Verification items for the finished model (mm, model axes). A direction names the side the tool comes from. Give positions to 0.01 mm unless a question says otherwise; leave off trailing zeros. Order: outer loops, then holes, each group sorted by start corner. A loop starts at its lowest first (then second) coordinate and runs counter-clockwise, first axis right, second up.
from build123d import *

# Parameters (mm, degrees)
BLOCK_BODY_DEPTH                       = 19.7
SIDE_REFERENCE_SKETCH_W                = 40
SIDE_REFERENCE_SKETCH_H                = 20
SIDE_REFERENCE_DEPTH                   = 0.45
AESTHETIC_CHAMFER_1_SIZE               = 0.5
CASTING_GROOVE_SKETCH_W                = 6
CASTING_GROOVE_SKETCH_H                = 40
CASTING_GOORVE_DEPTH                   = 0.75
AESTHETIC_CHAMFER_2_SIZE               = 0.2
PRODUCTION_FILLET_R                    = 0.2
FIXING_HOLES_D                         = 3.3
FIXING_HOLES_DEPTH                     = 7.1
FIXING_HOLES_CSINK_D                   = 4.2
FIXING_HOLES_CSINK_ANGLE               = 90
FIXING_HOLES_TIP                       = 0.991420021
END_CAP_FIXING_HOLES_FRONT_D           = 2.05
END_CAP_FIXING_HOLES_FRONT_DEPTH       = 6.35
END_CAP_FIXING_HOLES_FRONT_CSINK_D     = 2.7
END_CAP_FIXING_HOLES_FRONT_CSINK_ANGLE = 90
END_CAP_FIXING_HOLES_FRONT_TIP         = 0.615882135
END_CAP_FIXING_HOLES_BACK_D            = 2.05
END_CAP_FIXING_HOLES_BACK_DEPTH        = 6.35
END_CAP_FIXING_HOLES_BACK_CSINK_D      = 2.7
END_CAP_FIXING_HOLES_BACK_CSINK_ANGLE  = 90
END_CAP_FIXING_HOLES_BACK_TIP          = 0.615882135


with BuildPart() as part:
    # Block Profile → Block Body (new body, symmetric)
    with BuildSketch(Plane.XY):
        with BuildLine():
            Line((16, 4.3), (13, 4.3))
            Line((13, 4.3), (13, 8.2))
            ThreePointArc((13, 8.2), (12.970710678, 8.270710678), (12.9, 8.3))
            Line((12.9, 8.3), (4.85, 8.3))
            Line((4.85, 8.3), (4.85, 8.584314575))
            ThreePointArc((4.85, 8.584314575), (4.87283614, 8.699119605), (4.937867966, 8.796446609))
            Line((4.937867966, 8.796446609), (5.13367604, 8.992254684))
            ThreePointArc((5.13367604, 8.992254684), (5.223715255, 9.115101334), (5.272591987, 9.259356056))
            ThreePointArc((5.272591987, 9.259356056), (5.689339828, 10.060660172), (6.490643944, 10.477408013))
            ThreePointArc((6.490643944, 10.477408013), (6.766607459, 10.625414027), (6.900414725, 10.908534598))
            ThreePointArc((6.900414725, 10.908534598), (6.98601637, 11.08386098), (7.161342753, 11.169462626))
            ThreePointArc((7.161342753, 11.169462626), (7.474614052, 11.334529402), (7.6, 11.665685425))
            Line((7.6, 11.665685425), (7.6, 12.334314575))
            ThreePointArc((7.6, 12.334314575), (7.474614052, 12.665470598), (7.161342753, 12.830537374))
            ThreePointArc((7.161342753, 12.830537374), (6.98601637, 12.91613902), (6.900414725, 13.091465402))
            ThreePointArc((6.900414725, 13.091465402), (6.766607459, 13.374585973), (6.490643944, 13.522591987))
            ThreePointArc((6.490643944, 13.522591987), (5.689339828, 13.939339828), (5.272591987, 14.740643944))
            ThreePointArc((5.272591987, 14.740643944), (5.223715255, 14.884898666), (5.13367604, 15.007745316))
            Line((5.13367604, 15.007745316), (5.041421356, 15.1))
            Line((5.041421356, 15.1), (-5.041421356, 15.1))
            Line((-5.041421356, 15.1), (-5.13367604, 15.007745316))
            ThreePointArc((-5.13367604, 15.007745316), (-5.223715255, 14.884898666), (-5.272591987, 14.740643944))
            ThreePointArc((-5.272591987, 14.740643944), (-5.689339828, 13.939339828), (-6.490643944, 13.522591987))
            ThreePointArc((-6.490643944, 13.522591987), (-6.766607459, 13.374585973), (-6.900414725, 13.091465402))
            ThreePointArc((-6.900414725, 13.091465402), (-6.98601637, 12.91613902), (-7.161342753, 12.830537374))
            ThreePointArc((-7.161342753, 12.830537374), (-7.474614052, 12.665470598), (-7.6, 12.334314575))
            Line((-7.6, 12.334314575), (-7.6, 11.665685425))
            ThreePointArc((-7.6, 11.665685425), (-7.474614052, 11.334529402), (-7.161342753, 11.169462626))
            ThreePointArc((-7.161342753, 11.169462626), (-6.98601637, 11.08386098), (-6.900414725, 10.908534598))
            ThreePointArc((-6.900414725, 10.908534598), (-6.766607459, 10.625414027), (-6.490643944, 10.477408013))
            ThreePointArc((-6.490643944, 10.477408013), (-5.689339828, 10.060660172), (-5.272591987, 9.259356056))
            ThreePointArc((-5.272591987, 9.259356056), (-5.223715255, 9.115101334), (-5.13367604, 8.992254684))
            Line((-5.13367604, 8.992254684), (-4.937867966, 8.796446609))
            ThreePointArc((-4.937867966, 8.796446609), (-4.87283614, 8.699119605), (-4.85, 8.584314575))
            Line((-4.85, 8.584314575), (-4.85, 8.3))
            Line((-4.85, 8.3), (-12.9, 8.3))
            ThreePointArc((-12.9, 8.3), (-12.970710678, 8.270710678), (-13, 8.2))
            Line((-13, 8.2), (-13, 4.3))
            Line((-13, 4.3), (-16, 4.3))
            Line((-16, 4.3), (-17, 5.3))
            Line((-17, 5.3), (-17, 27))
            Line((-17, 27), (-16, 28))
            Line((-16, 28), (16, 28))
            Line((16, 28), (17, 27))
            Line((17, 27), (17, 5.3))
            Line((17, 5.3), (16, 4.3))
        make_face()
    extrude(amount=BLOCK_BODY_DEPTH, both=True)

    # Side Reference Sketch → Side Reference (cut)
    with BuildSketch(Plane(origin=(17, 0, 0), x_dir=(0, 0, -1), z_dir=(1, 0, 0))):
        with Locations((0, 12)):
            Rectangle(SIDE_REFERENCE_SKETCH_W, SIDE_REFERENCE_SKETCH_H)
    extrude(amount=-SIDE_REFERENCE_DEPTH, mode=Mode.SUBTRACT)

    # Aesthetic Chamfer 1
    aesthetic_chamfer_1_edges = [part.edges().sort_by_distance(p)[0] for p in [
        (-17, 16.15, -19.7),
        (-16.5, 27.5, -19.7),
        (0, 28, -19.7),
        (16.5, 27.5, -19.7),
        (17, 24.5, -19.7),
        (-17, 16.15, 19.7),
        (-16.5, 27.5, 19.7),
        (17, 24.5, 19.7),
        (16.5, 27.5, 19.7),
        (0, 28, 19.7),
    ]]
    chamfer(aesthetic_chamfer_1_edges, length=AESTHETIC_CHAMFER_1_SIZE)

    # Casting Groove Sketch → Casting Goorve (cut)
    with BuildSketch(Plane(origin=(0, 28, 0), x_dir=(1, 0, 0), z_dir=(0, 1, 0))):
        with Locations((-6, 0)):
            Rectangle(CASTING_GROOVE_SKETCH_W, CASTING_GROOVE_SKETCH_H)
        with Locations((6, 0)):
            Rectangle(CASTING_GROOVE_SKETCH_W, CASTING_GROOVE_SKETCH_H)
    extrude(amount=-CASTING_GOORVE_DEPTH, mode=Mode.SUBTRACT)

    # Aesthetic Chamfer 2
    aesthetic_chamfer_2_edges = [part.edges().sort_by_distance(p)[0] for p in [
        (17, 22, 0),
        (-9, 28, 0),
        (-3, 28, 0),
        (3, 28, 0),
        (9, 28, 0),
    ]]
    chamfer(aesthetic_chamfer_2_edges, length=AESTHETIC_CHAMFER_2_SIZE)

    # Production Fillet
    production_fillet_edges = [part.edges().sort_by_distance(p)[0] for p in [
        (16.55, 22, 0),
        (6, 27.25, -19.7),
        (-6, 27.25, -19.7),
        (-3, 27.375, -19.7),
        (-3, 27.375, 19.7),
        (-3, 27.25, 0),
        (-9, 27.375, -19.7),
        (-9, 27.25, 0),
        (-9, 27.375, 19.7),
        (-6, 27.25, 19.7),
        (9, 27.375, -19.7),
        (9, 27.375, 19.7),
        (9, 27.25, 0),
        (3, 27.375, -19.7),
        (3, 27.25, 0),
        (3, 27.375, 19.7),
        (6, 27.25, 19.7),
    ]]
    fillet(production_fillet_edges, radius=PRODUCTION_FILLET_R)

    # Fixing Holes
    with Locations(Plane(origin=(0, 28, 0), x_dir=(1, 0, 0), z_dir=(0, 1, 0))):
        with Locations((-13, -13), (-13, 13), (13, 13), (13, -13)):
            CounterSinkHole(FIXING_HOLES_D / 2, FIXING_HOLES_CSINK_D / 2, depth=FIXING_HOLES_DEPTH, counter_sink_angle=FIXING_HOLES_CSINK_ANGLE)
            with Locations((0, 0, -(FIXING_HOLES_DEPTH + FIXING_HOLES_TIP / 2))):  # 118° drill point
                Cone(0, FIXING_HOLES_D / 2, FIXING_HOLES_TIP, mode=Mode.SUBTRACT)

    # End Cap Fixing Holes Front
    with Locations(Plane.XY.offset(19.7)):
        with Locations((-11.5, 11.8), (11.5, 11.8)):
            CounterSinkHole(END_CAP_FIXING_HOLES_FRONT_D / 2, END_CAP_FIXING_HOLES_FRONT_CSINK_D / 2, depth=END_CAP_FIXING_HOLES_FRONT_DEPTH, counter_sink_angle=END_CAP_FIXING_HOLES_FRONT_CSINK_ANGLE)
            with Locations((0, 0, -(END_CAP_FIXING_HOLES_FRONT_DEPTH + END_CAP_FIXING_HOLES_FRONT_TIP / 2))):  # 118° drill point
                Cone(0, END_CAP_FIXING_HOLES_FRONT_D / 2, END_CAP_FIXING_HOLES_FRONT_TIP, mode=Mode.SUBTRACT)

    # End Cap Fixing Holes Back
    with Locations(Plane(origin=(0, 0, -19.7), x_dir=(-1, 0, 0), z_dir=(0, 0, -1))):
        with Locations((-11.5, 11.8), (11.5, 11.8)):
            CounterSinkHole(END_CAP_FIXING_HOLES_BACK_D / 2, END_CAP_FIXING_HOLES_BACK_CSINK_D / 2, depth=END_CAP_FIXING_HOLES_BACK_DEPTH, counter_sink_angle=END_CAP_FIXING_HOLES_BACK_CSINK_ANGLE)
            with Locations((0, 0, -(END_CAP_FIXING_HOLES_BACK_DEPTH + END_CAP_FIXING_HOLES_BACK_TIP / 2))):  # 118° drill point
                Cone(0, END_CAP_FIXING_HOLES_BACK_D / 2, END_CAP_FIXING_HOLES_BACK_TIP, mode=Mode.SUBTRACT)


solid = part.part
(1) Section check C-C, the plane z = 17. Give the number of separate pieces and of enclosed holes in the cut face, then the cut area to 3 significant figures.
Solved:
separate pieces: 1
enclosed holes: 2
area: 592 mm2
(2) Release check for a two-part mould opening along Y. For faces 1 (the conical face through (-11.36, 11.69, -12.84)), 2 (the flat face through (15, 4.3, 0)), 3 (the flat face through (-13, 6, 0)) record: pulls with the +Y half, pulls with the -Y half, needs draft (parallel to the pull), parting line crosses it, or undercut.
Solved:
face 1: undercut
face 2: pulls with the -Y half
face 3: needs draft
(3) Section check B-B, the plane x = -2. Enter the section's corners in (y, z).
Solved:
outline: (15.1, -19.7) - (27.5, -19.7) - (28, -19.2) - (28, 19.2) - (27.5, 19.7) - (15.1, 19.7) - close
(4) Go/stop test with flat-tipped pins: pin 1 (2 mm diameter, centred on y = 14, z = -3.5, fed in from +X); pin 2 (3 mm diameter, centred on x = 13, z = -13, fed in from +Y); pin 3 (2.5 mm diameter, centred on x = 11.5, y = 11.8, fed in from -Z). Record where each tip stops, or that it passes through.
Solved:
pin 1: stops at x = 16.55
pin 2: stops at y = 20.81
pin 3: stops at z = -19.6
(5) Section check A-A, the plane y = 23. Enter the section's corners in (x, z), then the cut area to 3 significant figures.
Solved:
outline: (-17, -19.2) - (-16.5, -19.7) - (16.5, -19.7) - (17, -19.2) - (17, 19.2) - (16.5, 19.7) - (-16.5, 19.7) - (-17, 19.2) - close; hole circle Ø3.3 at (-13, -13); hole circle Ø3.3 at (-13, 13); hole circle Ø3.3 at (13, -13); hole circle Ø3.3 at (13, 13)
area: 1,300 mm2
(6) Scan lines: line 1 (Z direction, x = 13, y = 25.5); line 2 (X direction, y = 11.8, z = 16.25) (3 decimals); line 3 (X direction, y = 23.5, z = -13). Record each from-to range of solid material in increasing order.
Solved:
line 1: z = -19.7 to -14.65, -11.35 to 11.35, 14.65 to 19.7
line 2: x = -17 to -12.525, -10.475 to -7.6, 7.6 to 10.475, 12.525 to 16.55
line 3: x = -17 to -14.65, -11.35 to 11.35, 14.65 to 17
(7) Set-up check for faces 4 (the flat face through (-6, 27.25, 0)), 5 (the flat face through (-9, 8.3, 0)), 6 (the cylindrical face through (-11.633, 12.816, -16.32)): record each of +Z, -Z, +X, -X, +Y, -Y from which the full face is reachable in a straight line by a thin tool's end or side.
Solved:
face 4: +Z, -Z, +Y
face 5: +Z, -Z, -Y
face 6: -Z
